The listing builds one solid part. Answer for the finished solid, in the listing's coordinates (mm). Coordinates: 2 decimals unless noted, no trailing zeros. Write each loop counter-clockwise with the first axis right and the second up, starting at its lowest first coordinate (ties: lowest second). Pieces come first, ordered by that corner, then holes.
(1) Given P1, Ø2.5, axis at x = 84.575, z = 0, coming from the +Y side, flat-ended and moving along its own axis, determine where the tip first touches the part or whether it passes through.
(2) The part is cut by section A-A on y = -0.45. Give the number of separate pieces and of enclosed holes in the cut face, plus the area to 3 significant figures.
(3) Straight lines are drawn through the part: line 1 (X direction, y = -0.2, z = -0.5); line 2 (X direction, y = -0.45, z = 0.75); line 3 (X direction, y = -0.7, z = 1.75). For each, find the intervals that lie inside material, in ascending order.
(4) The part is cut by section B-B on z = 5.25. Determine the outline of the cut face in (x, y), plus the area to 3 significant figures.
(5) For a pull along X with two mould halves and no side action, classify faces 1 (the cylindrical face through (-89.94, -0.44, 5.24)), 2 (the cylindrical face through (86.273, -0.436, -0.075)), 3 (the cylindrical face through (89.82, -0.44, 5.36)) as +X half, -X half, draft (parallel to the pull), parting line (faces both ways), or undercut.
from build123d import *

# Parameters (mm, degrees)
SKETCH2_W                = 184.15
SKETCH2_H                = 15
BASE_FLANGE1_DEPTH       = 0.86
M3_CLEARANCE_HOLE1_D     = 3.4
M3_CLEARANCE_HOLE1_DEPTH = 1.29
M3_CLEARANCE_HOLE1_TIP   = 1.021463052
FILLET1_R                = 7.5


# Sheet-metal steps are written as plain solids
with BuildPart() as part:
    # Sketch2 → Base-Flange1 (new body)
    with BuildSketch(Plane(origin=(0, 0, 0), x_dir=(1, 0, 0), z_dir=(0, 1, 0))):
        Rectangle(SKETCH2_W, SKETCH2_H)
    extrude(amount=-BASE_FLANGE1_DEPTH)

    # M3 Clearance Hole1
    with Locations(Plane(origin=(0, 0, 0), x_dir=(1, 0, 0), z_dir=(0, 1, 0))):
        with Locations((-84.575, 0), (84.575, 0)):
            Hole(M3_CLEARANCE_HOLE1_D / 2, depth=M3_CLEARANCE_HOLE1_DEPTH)
            with Locations((0, 0, -(M3_CLEARANCE_HOLE1_DEPTH + M3_CLEARANCE_HOLE1_TIP / 2))):  # 118° drill point
                Cone(0, M3_CLEARANCE_HOLE1_D / 2, M3_CLEARANCE_HOLE1_TIP, mode=Mode.SUBTRACT)

    # Fillet1
    fillet1_edges = [part.edges().sort_by_distance(p)[0] for p in [
        (92.075, -0.43, 7.5),
        (92.075, -0.43, -7.5),
        (-92.075, -0.43, 7.5),
        (-92.075, -0.43, -7.5),
    ]]
    fillet(fillet1_edges, radius=FILLET1_R - 0.0001)  # a hair under: the kernel refuses the full size


solid = part.part
Model answer:
1. P1: passes through
2. separate pieces: 1
2. enclosed holes: 2
2. area: 2,700 mm2
3. line 1: x = -92.06 to -86.2, -82.95 to 82.95, 86.2 to 92.06
3. line 2: x = -92.04 to -86.1, -83.05 to 83.05, 86.1 to 92.04
3. line 3: x = -91.87 to 91.87
4. outline: (-89.93, -0.86) - (89.93, -0.86) - (89.93, 0) - (-89.93, 0) - close
4. area: 155 mm2
5. face 1: -X half
5. face 2: undercut
5. face 3: +X half
